Check sheet for the modelled part. Datum: model origin and axes. Units: mm. A direction names the side the tool comes from. Give positions to 0.01 mm unless a question says otherwise; leave off trailing zeros. Order: outer loops, then holes, each group sorted by start corner. A loop starts at its lowest first (then second) coordinate and runs counter-clockwise, first axis right, second up.
Autodesk Inventor part; units mm, degrees
ref_plane "YZ Plane" through (0, 0, 0) normal (1, 0, 0) x (0, 1, 0)
ref_plane "XY Plane" through (0, 0, 0) normal (0, 0, 1) x (1, 0, 0)
sketch "Эскиз1" plane through (0, 0, 0) normal (0, 0, 1) x (1, 0, 0)
  circle A0 centre (0, 3) radius 3
  circle A1 centre (0, 3) radius 6
  point P0 (0, 0)
  dimension "d0" = 12
extrude "Выдавливание1" add sketch "Эскиз1" along normal blind 58
sketch "Эскиз2" plane through (0, 0, 0) normal (0, 1, 0) x (-1, 0, 0)
  line L0 (6, 58) -> (-6, 58)
  line L1 (0, 58) -> (0, 55) construction
  line L2 (0, 0) -> (0, 4.5)
  dimension "d4" = 3
  dimension "d5" = 4.5
ref_plane "РабПлоскость1" through (0, 2.25, 0) normal (0, 1, 0) x (-1, 0, 0)
sketch "Эскиз3" plane through (0, 2.25, 0) normal (0, 1, 0) x (-1, 0, 0)
  point P0 (0, 0)
  point P1 (0, 55)
  point P2 (0, 4.5)
hole "Отверстие1" at (0, 2.25, 55) at (0, 2.25, 4.5) direction (0, -1, 0) diameter 2.459 depth 8.8 tip angle 118
ref_plane "РабПлоскость2" through (0, 3, 52.5) normal (0, 0, 1) x (1, 0, 0)
sketch "Эскиз4" plane through (0, 3, 52.5) normal (0, 0, 1) x (1, 0, 0)
  circle A0 centre (0, 0) radius 5.65
  circle A1 centre (0, 0) radius 6.8955
  point P0 (0, -3)
  dimension "d15" = 11.3
extrude "Выдавливание2" cut sketch "Эскиз4" against normal blind 1.2
ref_plane "РабПлоскость3" through (0, 3, 8.5) normal (0, 0, -1) x (0.7866, 0.6175, 0)
sketch "Эскиз5" plane through (0, 3, 8.5) normal (0, 0, -1) x (0.7866, 0.6175, 0)
  circle A0 centre (0, 0) radius 5.65
  circle A1 centre (0, 0) radius 6.969
  point P0 (-1.8524, 2.3598)
  dimension "d18" = 11.3
extrude "Выдавливание3" cut sketch "Эскиз5" along normal blind 1.2
ref_plane "РабПлоскость4" through (6.468, -1.8388, 51.5) normal (-0.6175, 0.7866, 0) x (0.7866, 0.6175, 0)
sketch "Эскиз6" plane through (6.468, -1.8388, 51.5) normal (-0.6175, 0.7866, 0) x (0.7866, 0.6175, 0)
  line L0 (-8.1, -6.5) -> (3.9, -6.5)
  line L1 (-2.1, -6.5) -> (-2.1, 51.5) construction
  line L2 (-8.1, 51.5) -> (3.9, 51.5)
  line L3 (-2.1, 3.542) -> (-2.1, 39.542) construction
  line L4 (-0.1, 3.542) -> (-0.1, 39.542)
  line L5 (-4.1, 39.542) -> (-4.1, 3.542)
  arc A0 (-4.1, 3.542) -> (-0.1, 3.542) centre (-2.1, 3.542) ccw
  arc A1 (-0.1, 39.542) -> (-4.1, 39.542) centre (-2.1, 39.542) ccw
  point P0 (-3.9524, 51.5)
  point P1 (-2.1, 21.542)
  dimension "d21" = 36
  dimension "d22" = 4
extrude "Выдавливание4" cut sketch "Эскиз6" along normal blind 4.3
properties part number "Вал 2 оси"
(1) Go/stop test with flat-tipped pins: P1, Ø1, axis at x = -4, y = 0.5, coming from the -Z side; P2, Ø3, axis at x = 3, z = 19, coming from the -Y side; P3, Ø1.5, axis at x = 3, z = 19, coming from the -Y side. Record where each tip stops, or that it passes through.
(2) Thickness scan on L1, parallel to Z at x = -5.5, y = 4.75; L2, parallel to Z at x = 0, y = -2; L3, parallel to Y at x = 0, z = 39. Record the ranges inside material, lowest first.
(3) Sectioned sample at C-C (z = 19). Enter the section's corners in (x, y), plus the area to 3 significant figures.
(4) Sectioned sample at B-B (y = 3). Enter the section's corners in (x, z), plus the area to 3 significant figures.
(5) Tool access check on faces 1 (the face through (-1.301, 8.857, 29.6)), 2 (the face through (2.978, -0.722, 49.958)), 3 (the face through (1.262, -1.848, 29.706)), 4 (the face through (-0.05, -1.39, 53.77)). Record the directions out of +Z, -Z, +X, -X, +Y, -Y that give a thin tool (end or side, any length) a straight path to the whole face; none if there is none.
(6) Sectioned sample at D-D (y = 7.25). Enter the section's corners in (x, z), plus the area to 3 significant figures.
(7) Sectioned sample at A-A (x = 0). Count the separate pieces of the cut face and the enclosed holes in it, plus the area to 3 significant figures.
(8) Release check for a two-part mould opening along Y. For faces 5 (the face through (-3, 2, 58)), 6 (the face through (-0.65, 5.93, 28.59)), 7 (the face through (4.41, 0.62, 30.21)) record: released by +Y, released by -Y, zero draft, split by the parting line, or undercut.
Values follow:
1. P1: stops at z = 0
1. P2: stops at y = -2.81
1. P3: stops at y = 0.32
2. L1: z = 0 to 7.3, 8.5 to 51.3, 52.5 to 58
2. L2: z = 0 to 3.27, 5.73 to 53.77, 56.23 to 58
2. L3: y = -3 to 0, 6 to 9
3. outline: (0.59, -0.99) - (3.73, 1.48) - (5.07, -0.21) arc R6 ccw (long way) to (1.92, -2.68) - close; hole circle Ø6 at (0, 3)
3. area: 75.3 mm2
4. outline: (-6, 0) - (-3, 0) - (-3, 58) - (-6, 58) - (-6, 52.5) - (-5.65, 52.5) - (-5.65, 51.3) - (-6, 51.3) - (-6, 8.5) - (-5.65, 8.5) - (-5.65, 7.3) - (-6, 7.3) - close; (3, 0) - (6, 0) - (6, 7.3) - (5.65, 7.3) - (5.65, 8.5) - (6, 8.5) - (6, 51.3) - (5.65, 51.3) - (5.65, 52.5) - (6, 52.5) - (6, 58) - (3, 58) - close
4. area: 346 mm2
5. face 1: +Z, -Z
5. face 2: none
5. face 3: +X
5. face 4: -Y
6. outline: (-4.24, 0) - (4.24, 0) - (4.24, 7.3) - (3.72, 7.3) - (3.72, 8.5) - (4.24, 8.5) - (4.24, 51.3) - (3.72, 51.3) - (3.72, 52.5) - (4.24, 52.5) - (4.24, 58) - (-4.24, 58) - (-4.24, 52.5) - (-3.72, 52.5) - (-3.72, 51.3) - (-4.24, 51.3) - (-4.24, 8.5) - (-3.72, 8.5) - (-3.72, 7.3) - (-4.24, 7.3) - close
6. area: 489 mm2
7. separate pieces: 4
7. enclosed holes: 0
7. area: 332 mm2
8. face 5: zero draft
8. face 6: undercut
8. face 7: released by -Y
